Read the model definition and answer for the solid it produces. Units are mm, in the model's axes. Face numbers are marked on the shaded views. A direction names the side the tool comes from. Round coordinates to 2 decimals unless told otherwise and drop trailing zeros. Order: outer loops, then holes, each group sorted by start corner. A loop starts at its lowest first (then second) coordinate and runs counter-clockwise, first axis right, second up. Notation, with made-up numbers: (-19.5, 38) -> (7.5, 38) arc R18 cw to (7.5, 68) -> close; hole circle Ø3 at (-27.5, 81). An arc over 180 degrees is marked (long way). Use a Markdown table: item, result. Add a question column.
1. Given pin 1 (3 mm diameter, centred on x = -5, y = -6.5, fed in from -Z); pin 2 (6 mm diameter, centred on y = 4, z = -0.5, fed in from +X); pin 3 (5 mm diameter, centred on x = 3.5, z = -7, fed in from -Y), each flat-ended and moving along its own axis, determine where each tip first touches the part or whether it passes through.
2. Section C-C, the plane z = -23 is taken. Give the vertices of the cut face in (x, y), then the cut area to 3 significant figures.
3. For the marked faces 1, 2 and 3, determine the directions among +Z, -Z, +X, -X, +Y, -Y from which every point of the face is accessible in a straight line to the end or side of a thin tool.
4. Consider L1, parallel to Z at x = -6.5, y = 1.25; L2, parallel to Y at x = 0.25, z = -18; L3, parallel to Y at x = 0, z = -23. Determine where each line is inside the solid, lowest interval first. Write a range as [from, to].
5. Section D-D, the plane z = 12 is taken. Give the vertices of the cut face in (x, y) (3 decimals), then the cut area to 3 significant figures.
6. Section A-A, the plane x = 0 is taken. Give the vertices of the cut face in (y, z) (3 decimals), then the cut area to 3 significant figures.
```python
from build123d import *


with BuildPart() as part:
    # Sketch1 → Base-Revolve (revolve)
    with BuildSketch(Plane(origin=(0, 0, 0), x_dir=(0, 0, -1), z_dir=(1, 0, 0)), mode=Mode.PRIVATE) as base_revolve_sk:
        Polygon((-40, 0), (-40, 5.90625), (-20, 5.90625), (-20, 7.875), (20, 7.875), (20, 5.90625), (40, 5.90625), (40, 0), align=None)
    revolve(base_revolve_sk.sketch.rotate(Axis((0, 0, 61.5315), (0, 0, -1)), 90), axis=Axis((0, 0, 61.5315), (0, 0, -1)))


solid = part.part
```
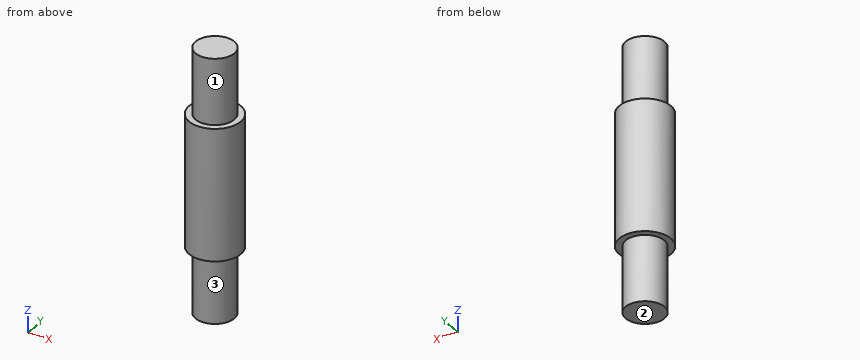
Verdict:
| question | item | result |
|---|---|---|
| 1 | pin 1 | stops at z = -20 |
| 1 | pin 2 | stops at x = 7.81 |
| 1 | pin 3 | stops at y = -7.81 |
| 2 | outline | circle Ø11.81 at (0, 0) |
| 2 | area | 110 mm2 |
| 3 | face 1 | +Z |
| 3 | face 2 | -Z, +X, -X, +Y, -Y |
| 3 | face 3 | -Z |
| 4 | L1 | z = [-20, 20] |
| 4 | L2 | y = [-7.87, 7.87] |
| 4 | L3 | y = [-5.91, 5.91] |
| 5 | outline | circle Ø15.75 at (0, 0) |
| 5 | area | 195 mm2 |
| 6 | outline | (-7.875, -20) -> (-5.906, -20) -> (-5.906, -40) -> (5.906, -40) -> (5.906, -20) -> (7.875, -20) -> (7.875, 20) -> (5.906, 20) -> (5.906, 40) -> (-5.906, 40) -> (-5.906, 20) -> (-7.875, 20) -> close |
| 6 | area | 1,100 mm2 |
